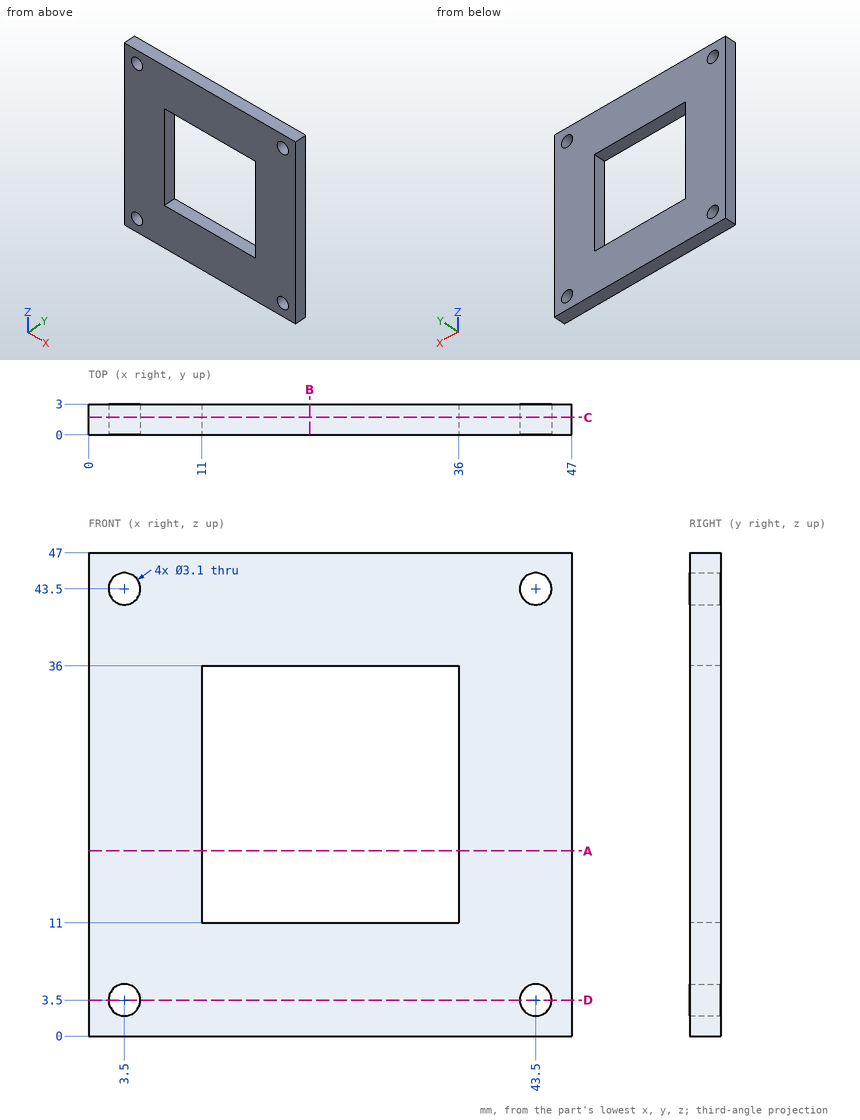
Part print with two shaded views. Sizes in mm from the minimum x, y, z corner. Give positions to 0.01 mm unless a question says otherwise; leave off trailing zeros. Order: outer loops, then holes, each group sorted by start corner. A loop starts at its lowest first (then second) coordinate and runs counter-clockwise, first axis right, second up. Notation, with made-up numbers: (13, 17) - (29, 17) arc R9 cw to (29, 26) - close; hole circle Ø10 at (3, 4). An arc over 180 degrees is marked (long way). Write each question's results on one line, items separated by ' | '.
1. Saw through at A-A on z = 18. List the corners of the cut face in (x, y), and give its area (3 significant figures).
Calculated:
outline: (0, 0) - (11, 0) - (11, 3) - (0, 3) - close; (36, 0) - (47, 0) - (47, 3) - (36, 3) - close | area: 66.0 mm2
2. Pin check, flat tip, straight feed: pin 1 (3 mm diameter, centred on x = 43.5, z = 3.5, fed in from +Y). Stop position of the tip, or through.
Calculated:
pin 1: passes through
3. Saw through at C-C on y = 1.7. List the corners of the cut face in (x, z).
Calculated:
outline: (0, 0) - (47, 0) - (47, 47) - (0, 47) - close; hole circle Ø3.1 at (3.5, 3.5); hole circle Ø3.1 at (3.5, 43.5); hole (11, 11) - (36, 11) - (36, 36) - (11, 36) - close; hole circle Ø3.1 at (43.5, 3.5); hole circle Ø3.1 at (43.5, 43.5)
4. Saw through at B-B on x = 21.5. List the corners of the cut face in (y, z).
Calculated:
outline: (0, 0) - (3, 0) - (3, 11) - (0, 11) - close; (0, 36) - (3, 36) - (3, 47) - (0, 47) - close
5. Probe L1, parallel to X at y = 1.9, z = 43.5; L2, parallel to X at y = 1.9, z = 16.5. List the from-to ranges inside material, lowest first. Write a range as from..to.
Calculated:
L1: x = 0..1.95, 5.05..41.95, 45.05..47 | L2: x = 0..11, 36..47
6. Saw through at D-D on z = 3.5. List the corners of the cut face in (x, y), and give its area (3 significant figures).
Calculated:
outline: (0, 0) - (1.95, 0) - (1.95, 3) - (0, 3) - close; (5.05, 0) - (41.95, 0) - (41.95, 3) - (5.05, 3) - close; (45.05, 0) - (47, 0) - (47, 3) - (45.05, 3) - close | area: 122 mm2
